Here's how the part is built. I have some questions about the finished solid (model axes, mm). A direction names the side the tool comes from. Coordinates: 2 decimals unless noted, no trailing zeros. Write each loop counter-clockwise with the first axis right and the second up, starting at its lowest first coordinate (ties: lowest second). Pieces come first, ordered by that corner, then holes. Notation, with made-up numbers: (23, 80.5) -> (40, 80.5) arc R17 ccw to (40, 110.5) -> close; hole circle Ø8 at (63, 37.25). An arc over 180 degrees is marked (long way). Put each result on its own line as item: value.
Autodesk Inventor part; units mm, degrees
ref_plane "ANSCHRAUB_XY" through (0, 0, 145) normal (0, 0, 1) x (1, 0, 0)
ref_plane "ANSCHRAUB_YZ" through (0, 0, 145) normal (1, 0, 0) x (0, 1, 0)
ref_plane "ANSCHRAUB_ZX" through (0, 0, 145) normal (0, 1, 0) x (0, 0, 1)
sketch "Base_KS" plane through (0, 0, 0) normal (1, 0, 0) x (0, 1, 0)
  line L0 (0, 0) -> (0, 122.9)
  line L1 (0, 122.9) -> (3, 122.9)
  line L2 (3, 122.9) -> (3, 6)
  line L3 (3, 6) -> (16, 6)
  line L4 (16, 6) -> (16, 0)
  line L5 (16, 0) -> (0, 0)
  line L6 (0, 0) -> (0, 122.9)
revolve "Revolution1" add sketch "Base_KS" angle 360 about axis through (0, 0, 0) along (0, 0, -1)
sketch "Skizze_2" plane through (0, 0, 0) normal (1, 0, 0) x (0, 1, 0)
  line L0 (0, 0.1) -> (0, 123)
  line L1 (0, 123) -> (6, 123)
  line L2 (6, 123) -> (6, 0.1)
  line L3 (6, 0.1) -> (0, 0.1)
  line L4 (0, 0.1) -> (0, 123)
revolve "Revolution2" add sketch "Skizze_2" angle 360 about axis through (0, 0, 0.1) along (0, 0, -1)
sketch "Skizze_4" plane through (0, 0, 123) normal (0, 0, 1) x (0, 1, 0)
  line L0 (5, 12) -> (5, -12)
  line L1 (5, -12) -> (12, -12)
  line L2 (12, -12) -> (12, 12)
  line L3 (12, 12) -> (5, 12)
extrude "Extrusion1" cut sketch "Skizze_4" along normal mid plane 10
sketch "Skizze_5" plane through (0, 0, 123) normal (0, 0, 1) x (0, 1, 0)
  line L0 (-12, 12) -> (-12, -12)
  line L1 (-12, -12) -> (-5, -12)
  line L2 (-5, -12) -> (-5, 12)
  line L3 (-5, 12) -> (-12, 12)
extrude "Extrusion2" cut sketch "Skizze_5" along normal mid plane 10
sketch "Skizze_8" plane through (0, 0, 0) normal (1, 0, 0) x (0, 1, 0)
  line L0 (0, 122.9) -> (0, 145)
  line L1 (0, 145) -> (4.233, 145)
  line L2 (4.233, 145) -> (5, 144.233)
  line L3 (5, 144.233) -> (5, 123.667)
  line L4 (5, 123.667) -> (4.233, 122.9)
  line L5 (4.233, 122.9) -> (0, 122.9)
  line L6 (0, 122.9) -> (0, 145)
revolve "Revolution3" add sketch "Skizze_8" angle 360 about axis through (0, 0, 122.9) along (0, 0, -1)
thread "Thread1"
ref_plane "ANSCHRAUB_XY" through (0, 0, 145) normal (0, 0, 1) x (1, 0, 0)
ref_plane "ANSCHRAUB_YZ" through (0, 0, 145) normal (1, 0, 0) x (0, 1, 0)
ref_plane "ANSCHRAUB_ZX" through (0, 0, 145) normal (0, 1, 0) x (0, 0, 1)
ref_plane "CP_30_XY" through (0, 0, 123) normal (0, 0, 1) x (1, 0, 0)
ref_plane "CP_30_YZ" through (0, 0, 123) normal (1, 0, 0) x (0, 1, 0)
ref_plane "CP_30_ZX" through (0, 0, 123) normal (0, 1, 0) x (0, 0, 1)
ref_plane "KS_AUFSATZ1_XY" through (0, 0, 132) normal (0, 0, 1) x (1, 0, 0)
ref_plane "KS_AUFSATZ1_YZ" through (0, 0, 132) normal (1, 0, 0) x (0, 1, 0)
ref_plane "KS_AUFSATZ1_ZX" through (0, 0, 132) normal (0, 1, 0) x (0, 0, 1)
ref_plane "NUT1_XY" through (0, 0, 132) normal (0, 0, -1) x (1, 0, 0)
ref_plane "NUT1_YZ" through (0, 0, 132) normal (1, 0, 0) x (0, -1, 0)
ref_plane "NUT1_ZX" through (0, 0, 132) normal (0, -1, 0) x (0, 0, -1)
ref_plane "ZYLINDER_XY" through (0, 0, 0) normal (0, 0, 1) x (1, 0, 0)
ref_plane "ZYLINDER_YZ" through (0, 0, 0) normal (1, 0, 0) x (0, 1, 0)
ref_plane "ZYLINDER_ZX" through (0, 0, 0) normal (0, 1, 0) x (0, 0, 1)
properties part number "DNC-32-50---(KS)"
Item 1: Imagine slicing it at A-A on x = -10. Write out the boundary of the cut face in (y, z).
Output:
outline: (-12.49, 0) -> (12.49, 0) -> (12.49, 6) -> (-12.49, 6) -> close
Item 2: Imagine slicing it at B-B on y = 0. Write out the boundary of the cut face in (x, z).
Output:
outline: (-16, 0) -> (16, 0) -> (16, 6) -> (6, 6) -> (6, 123) -> (4.33, 123) -> (5, 123.67) -> (5, 144.23) -> (4.23, 145) -> (-4.23, 145) -> (-5, 144.23) -> (-5, 123.67) -> (-4.33, 123) -> (-6, 123) -> (-6, 6) -> (-16, 6) -> close
Item 3: If we mould it in two halves opening along Z, with no side actions, what happens to faces 1 (the flat face through (0, 5, 120)), 2 (the flat face through (0, 0, 0)), 3 (the flat face through (-1.2, 4.4, 123))? For each: released by +Z, released by -Z, zero draft, split by the parting line, or undercut.
Output:
face 1: zero draft
face 2: released by -Z
face 3: undercut
Item 4: Imagine slicing it at D-D on x = 0. Write out the boundary of the cut face in (y, z), then the cut area to 3 significant figures.
Output:
outline: (-16, 0) -> (16, 0) -> (16, 6) -> (6, 6) -> (6, 118) -> (5, 118) -> (5, 123) -> (4.33, 123) -> (5, 123.67) -> (5, 144.23) -> (4.23, 145) -> (-4.23, 145) -> (-5, 144.23) -> (-5, 123.67) -> (-4.33, 123) -> (-5, 123) -> (-5, 118) -> (-6, 118) -> (-6, 6) -> (-16, 6) -> close
area: 1,800 mm²
Item 5: For P1, Ø1, axis at x = -1, z = 127, coming from the -Y side; P2, Ø5, axis at y = -6, z = 41, coming from the -X side; P3, Ø4, axis at x = 3, z = 93, coming from the -Y side, each with a flat end and sliding along its axis, tell me the tip position at first contact or that it passes through.
Output:
P1: stops at y = -4.97
P2: stops at x = -4.87
P3: stops at y = -5.92
Item 6: Which directions (+Z, -Z, +X, -X, +Y, -Y) give clear straight access to the entire face, cutting with the end or side of a thin tool? Please do faces 4 (the flat face through (0, -5, 120)), 5 (the cylindrical face through (-4.88, -1.08, 133.81)), 6 (the cylindrical face through (-15.62, -3.47, 2.96)).
Output:
face 4: +Z, +X, -X, -Y
face 5: +Z
face 6: +Z, -Z
Item 7: Please list where these lines run through material, in increasing order: line 1 along Z through (x, y) = (9.5, 5); line 2 along Y through (x, z) = (0.5, 21.5); line 3 along X through (y, z) = (-3, 11.5). Write a range as from..to.
Output:
line 1: z = 0..6
line 2: y = -5.98..5.98
line 3: x = -5.2..5.2
Item 8: Imagine slicing it at C-C on z = 79. Write out the boundary of the cut face in (x, y).
Output:
outline: circle Ø12 at (0, 0)
